```python
from build123d import *

# Parameters (mm, degrees)
F0_R     = 11
F1_DEPTH = 8


with BuildPart() as f1:
    # F0 (on Top) → F1 (new body)
    with BuildSketch(Plane.XY):
        with BuildLine():
            ThreePointArc((-10.781154, 8.931222), (0, 14), (10.781154, 8.931222))
            ThreePointArc((10.781154, 8.931222), (10.950081, 12.071765), (11.730086, 15.11859))
            ThreePointArc((11.730086, 15.11859), (13.112032, 17.988443), (15.035082, 20.527678))
            ThreePointArc((15.035082, 20.527678), (13.221629, 23.66867), (16, 26))
            ThreePointArc((16, 26), (15.756924, 28.778371), (15.035082, 31.472322))
            ThreePointArc((15.035082, 31.472322), (11.626906, 32.712797), (12.256711, 36.284602))
            ThreePointArc((12.256711, 36.284602), (10.284602, 38.256711), (8, 39.856406))
            ThreePointArc((8, 39.856406), (4.591824, 38.615932), (2.778371, 41.756924))
            ThreePointArc((2.778371, 41.756924), (0, 42), (-2.778371, 41.756924))
            ThreePointArc((-2.778371, 41.756924), (-4.591824, 38.615932), (-8, 39.856406))
            ThreePointArc((-8, 39.856406), (-10.284602, 38.256711), (-12.256711, 36.284602))
            ThreePointArc((-12.256711, 36.284602), (-11.626906, 32.712797), (-15.035082, 31.472322))
            ThreePointArc((-15.035082, 31.472322), (-15.756924, 28.778371), (-16, 26))
            ThreePointArc((-16, 26), (-13.221629, 23.66867), (-15.035082, 20.527678))
            ThreePointArc((-15.035082, 20.527678), (-13.112032, 17.988443), (-11.730086, 15.11859))
            ThreePointArc((-11.730086, 15.11859), (-10.950081, 12.071765), (-10.781154, 8.931222))
        make_face()
        with Locations((0, 26)):
            Circle(F0_R, mode=Mode.SUBTRACT)
        with BuildLine():
            ThreePointArc((10.781154, -8.931222), (13.170728, -4.74678), (14, 0))
            ThreePointArc((14, 0), (13.170728, 4.74678), (10.781154, 8.931222))
            ThreePointArc((10.781154, 8.931222), (0, 14), (-10.781154, 8.931222))
            ThreePointArc((-10.781154, 8.931222), (-14, 0), (-10.781154, -8.931222))
            ThreePointArc((-10.781154, -8.931222), (0, -14), (10.781154, -8.931222))
        make_face()
        Circle(F0_R, mode=Mode.SUBTRACT)
        with BuildLine():
            ThreePointArc((11.730086, -15.11859), (10.950081, -12.071765), (10.781154, -8.931222))
            ThreePointArc((10.781154, -8.931222), (0, -14), (-10.781154, -8.931222))
            ThreePointArc((-10.781154, -8.931222), (-10.950081, -12.071765), (-11.730086, -15.11859))
            ThreePointArc((-11.730086, -15.11859), (-13.112032, -17.988443), (-15.035082, -20.527678))
            ThreePointArc((-15.035082, -20.527678), (-13.221629, -23.66867), (-16, -26))
            ThreePointArc((-16, -26), (-15.756924, -28.778371), (-15.035082, -31.472322))
            ThreePointArc((-15.035082, -31.472322), (-11.626906, -32.712797), (-12.256711, -36.284602))
            ThreePointArc((-12.256711, -36.284602), (-10.284602, -38.256711), (-8, -39.856406))
            ThreePointArc((-8, -39.856406), (-4.591824, -38.615932), (-2.778371, -41.756924))
            ThreePointArc((-2.778371, -41.756924), (0, -42), (2.778371, -41.756924))
            ThreePointArc((2.778371, -41.756924), (4.591824, -38.615932), (8, -39.856406))
            ThreePointArc((8, -39.856406), (10.284602, -38.256711), (12.256711, -36.284602))
            ThreePointArc((12.256711, -36.284602), (11.626906, -32.712797), (15.035082, -31.472322))
            ThreePointArc((15.035082, -31.472322), (15.756924, -28.778371), (16, -26))
            ThreePointArc((16, -26), (13.221629, -23.66867), (15.035082, -20.527678))
            ThreePointArc((15.035082, -20.527678), (13.112032, -17.988443), (11.730086, -15.11859))
        make_face()
        with Locations((0, -26)):
            Circle(F0_R, mode=Mode.SUBTRACT)
    extrude(amount=F1_DEPTH)


solid = f1.part
```
Input: part model. Units: mm. Frame: model coordinates. A direction names the side the tool comes from. Give positions to 0.01 mm unless a question says otherwise; leave off trailing zeros. Order: outer loops, then holes, each group sorted by start corner. A loop starts at its lowest first (then second) coordinate and runs counter-clockwise, first axis right, second up.
1. Reachability of faces 4 (the cylindrical face through (13.09, 17.95, 3.94)), 5 (the cylindrical face through (-13.135, 18.027, 3.944)), 6 (the cylindrical face through (-2.38, 15.26, 3.94)) from +Z, -Z, +X, -X, +Y, -Y: full face, straight path, thin tool, end or side. Return the list, or none.
Derived:
face 4: +Z, -Z, +X
face 5: +Z, -Z, -X
face 6: +Z, -Z
2. Section B-B on y = -6.5. Return the cut outline in (x, z), and give its area (3 significant figures).
Derived:
outline: (-12.4, 0) - (-8.87, 0) - (-8.87, 8) - (-12.4, 8) - close; (8.87, 0) - (12.4, 0) - (12.4, 8) - (8.87, 8) - close
area: 56.4 mm2
3. Section D-D on y = 7. Return the cut outline in (x, z).
Derived:
outline: (-12.12, 0) - (-8.49, 0) - (-8.49, 8) - (-12.12, 8) - close; (8.49, 0) - (12.12, 0) - (12.12, 8) - (8.49, 8) - close
4. Section C-C on z = 4.5. Give the number of separate pieces and of enclosed holes in the cut face, and give its area (3 significant figures).
Derived:
separate pieces: 1
enclosed holes: 3
area: 901 mm2
5. Pin query (flat end, axial travel): pin 1 (17.5 mm diameter, centred on x = 0, y = 0, fed in from +Z); pin 2 (3 mm diameter, centred on y = 16, z = 5.5, fed in from -X). Return the tip coordinate at first contact, or that it passes through.
Derived:
pin 1: passes through
pin 2: stops at x = -12.83
6. Material intervals for L1, parallel to Y at x = 0, z = 2.5; L2, parallel to Y at x = 4, z = 4.75; L3, parallel to Y at x = -13, z = 7.5, sorted ascending.
Derived:
L1: y = -42 to -37, -15 to -11, 11 to 15, 37 to 42
L2: y = -38.91 to -36.25, -15.75 to -10.25, 10.25 to 15.75, 36.25 to 38.91
L3: y = -31.51 to -17.8, -5.2 to 5.2, 17.8 to 31.51
7. Section A-A on x = 0. Return the cut outline in (y, z), and give its area (3 significant figures).
Derived:
outline: (-42, 0) - (-37, 0) - (-37, 8) - (-42, 8) - close; (-15, 0) - (-11, 0) - (-11, 8) - (-15, 8) - close; (11, 0) - (15, 0) - (15, 8) - (11, 8) - close; (37, 0) - (42, 0) - (42, 8) - (37, 8) - close
area: 144 mm2
8. Mould query, pull axis Y, two halves, no side actions, for faces 1 (the flat face through (-7, -9, 0)), 2 (the cylindrical face through (-2.38, -36.74, 3.94)), 3 (the cylindrical face through (-10.255, 38.282, 3.944)). Classes: released by +Y, released by -Y, zero draft, split by the parting line, or undercut.
Derived:
face 1: zero draft
face 2: undercut
face 3: released by +Y
